Here's how the part is built. I have some questions about the finished solid (model axes, mm). Face numbers are marked on the shaded views. A direction names the side the tool comes from. Coordinates: 2 decimals unless noted, no trailing zeros. Write each loop counter-clockwise with the first axis right and the second up, starting at its lowest first coordinate (ties: lowest second). Pieces come first, ordered by that corner, then holes.
Item 1: If we mould it in two halves opening along Z, with no side actions, what happens to the marked faces 3, 4 and 5? For each: pulls with the +Z half, pulls with the -Z half, needs draft (parallel to the pull), parting line crosses it, or undercut.
Item 2: I want a section at A-A (y = 22.5). Please give me the cut outline in (x, z).
Item 3: Please list where these lines run through material, in increasing order: line 1 (X direction, y = 0.3, z = 0); line 2 (X direction, y = 67.8, z = 0); line 3 (Y direction, x = -4, z = 2).
Item 4: I'm going to push flat-ended pins straight in: P1, Ø4, axis at y = 48.5, z = -5.5, coming from the -X side; P2, Ø1.5, axis at x = -1, y = 10, coming from the -Z side; P3, Ø10, axis at x = -1.5, y = 49, coming from the +Z side; P4, Ø1, axis at x = 4.5, y = 37.5, coming from the +Z side. Where does each tip first touch, or does it pass through?
Item 5: For the marked faces 1 and 2, which set-ups out of +Z, -Z, +X, -X, +Y, -Y let a thin tool reach every point of the face, with its end or its side?
from build123d import *

# Parameters (mm, degrees)
SZKIC1_R                    = 9.35
DODANIE_WYCI_GNI_CIE1_DEPTH = 68.2
SZKIC2_R                    = 7
WYTNIJ_WYCI_GNI_CIE1_DEPTH  = 0.5
SZKIC3_R                    = 6
WYTNIJ_WYCI_GNI_CIE2_DEPTH  = 0.5
SZKIC4_R                    = 3
DODANIE_WYCI_GNI_CIE2_DEPTH = 1
ZAOKR_GLENIE1_R             = 0.5
SFAZOWANIE1_SIZE            = 0.5
SFAZOWANIE1_SIZE2           = 0.866025404


with BuildPart() as part:
    # Szkic1 → Dodanie-wyciągnięcie1 (new body)
    with BuildSketch(Plane(origin=(0, 0, 0), x_dir=(1, 0, 0), z_dir=(0, 1, 0))):
        with Locations(Location((0, 0, 0), (0, 0, 270))):
            Circle(SZKIC1_R)
    extrude(amount=DODANIE_WYCI_GNI_CIE1_DEPTH)

    # Szkic2 → Wytnij-wyciągnięcie1 (cut)
    with BuildSketch(Plane.XZ):
        with Locations(Location((0, 0, 0), (0, 0, 270))):
            Circle(SZKIC2_R)
    extrude(amount=-WYTNIJ_WYCI_GNI_CIE1_DEPTH, mode=Mode.SUBTRACT)

    # Szkic3 → Wytnij-wyciągnięcie2 (cut)
    with BuildSketch(Plane(origin=(0, 68.2, 0), x_dir=(1, 0, 0), z_dir=(0, 1, 0))):
        with Locations(Location((0, 0, 0), (0, 0, 270))):
            Circle(SZKIC3_R)
    extrude(amount=-WYTNIJ_WYCI_GNI_CIE2_DEPTH, mode=Mode.SUBTRACT)

    # Szkic4 → Dodanie-wyciągnięcie2 (add)
    with BuildSketch(Plane(origin=(0, 67.7, 0), x_dir=(1, 0, 0), z_dir=(0, 1, 0))):
        with Locations(Location((0, 0, 0), (0, 0, 270))):
            Circle(SZKIC4_R)
    extrude(amount=DODANIE_WYCI_GNI_CIE2_DEPTH)

    # Zaokrąglenie1
    zaokr_glenie1_edges = [part.edges().sort_by_distance(p)[0] for p in [
        (0, 68.7, -3),
    ]]
    fillet(zaokr_glenie1_edges, radius=ZAOKR_GLENIE1_R)

    # Sfazowanie1
    sfazowanie1_edges = [part.edges().sort_by_distance(p)[0] for p in [
        (0, 68.2, -9.35),
    ]]
    sfazowanie1_side = [part.faces().sort_by_distance(p)[0] for p in [
        (0, 68.2, -9.085542064),
    ]]
    chamfer(sfazowanie1_edges, length=SFAZOWANIE1_SIZE, length2=SFAZOWANIE1_SIZE2, reference=sfazowanie1_side[0])


solid = part.part
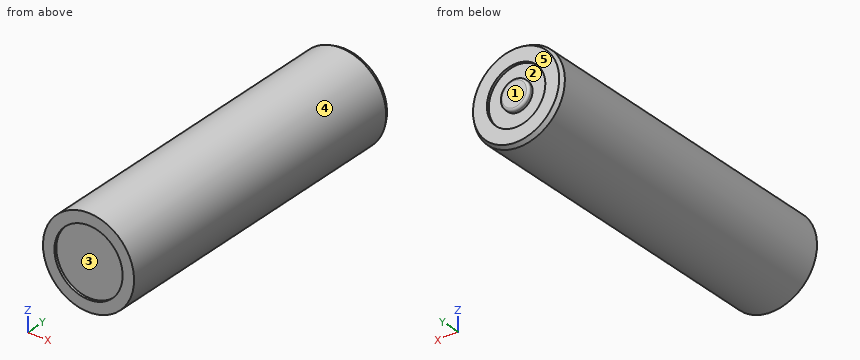
Answer:
1. face 3: undercut
1. face 4: parting line crosses it
1. face 5: needs draft
2. outline: circle Ø18.7 at (0, 0)
3. line 1: x = -9.35 to -7, 7 to 9.35
3. line 2: x = -9.08 to -6, -3 to 3, 6 to 9.08
3. line 3: y = 0.5 to 67.7
4. P1: stops at x = -8.67
4. P2: stops at z = -9.35
4. P3: stops at z = 9.35
4. P4: stops at z = 8.45
5. face 1: +Z, -Z, +X, -X, +Y
5. face 2: +Y
